from build123d import *

# Parameters (mm, degrees)
BOSS_EXTRUDE1_DEPTH = 3.175
CUT_EXTRUDE1_DEPTH  = 204.138678001
SKETCH3_W           = 42
SKETCH3_H           = 55.35
SKETCH3_W_2         = 7.65
SKETCH3_H_2         = 6.35
CUT_EXTRUDE2_DEPTH  = 204.138678001
SKETCH5_R           = 2
CUT_EXTRUDE4_DEPTH  = 204.138678001


with BuildPart() as part:
    # Sketch1 → Boss-Extrude1 (new, symmetric)
    with BuildSketch(Plane(origin=(0, 0, 0), x_dir=(1, 0, 0), z_dir=(0, 1, 0))):
        with BuildLine():
            Line((35, -200), (35, 0))
            ThreePointArc((35, 0), (0, 35), (-35, 0))
            Line((-35, 0), (-35, -200))
            Line((-35, -200), (35, -200))
        make_face()
    extrude(amount=BOSS_EXTRUDE1_DEPTH, both=True)

    # Sketch2 → Cut-Extrude1 (cut, through all)
    with BuildSketch(Plane(origin=(0, 3.175, 0), x_dir=(1, 0, 0), z_dir=(0, 1, 0))):
        with BuildLine():
            Line((-35, -38), (35, -38))
            Line((35, -38), (35, 0))
            ThreePointArc((35, 0), (0, 35), (-35, 0))
            Line((-35, 0), (-35, -38))
        make_face()
    extrude(amount=-CUT_EXTRUDE1_DEPTH, mode=Mode.SUBTRACT)

    # Sketch3 → Cut-Extrude2 (cut, through all)
    with BuildSketch(Plane(origin=(0, 3.175, 0), x_dir=(1, 0, 0), z_dir=(0, 1, 0))):
        with Locations((0, -87.325)):
            Rectangle(SKETCH3_W, SKETCH3_H)
        with Locations((-24.825, -111.825)):
            Rectangle(SKETCH3_W_2, SKETCH3_H_2)
        with Locations((24.825, -111.825)):
            Rectangle(SKETCH3_W_2, SKETCH3_H_2)
    extrude(amount=-CUT_EXTRUDE2_DEPTH, mode=Mode.SUBTRACT)

    # Sketch5 → Cut-Extrude4 (cut, through all)
    with BuildSketch(Plane(origin=(0, 3.175, 0), x_dir=(1, 0, 0), z_dir=(0, 1, 0))):
        with Locations(Location((27.5, -195.35, 0), (0, 0, 270))):
            Circle(SKETCH5_R)
        with Locations(Location((-27.5, -195.35, 0), (0, 0, 270))):
            Circle(SKETCH5_R)
        with Locations((15, -65.35)):
            Circle(SKETCH5_R)
        with Locations((-15, -65.35)):
            Circle(SKETCH5_R)
    extrude(amount=-CUT_EXTRUDE4_DEPTH, mode=Mode.SUBTRACT)


solid = part.part
Could you check a few things on this model? Use its own coordinates, in mm. A direction names the side the tool comes from. Give positions to 0.01 mm unless a question says otherwise; leave off trailing zeros. Write each loop counter-clockwise with the first axis right and the second up, starting at its lowest first coordinate (ties: lowest second). Pieces come first, ordered by that corner, then holes. Notation, with made-up numbers: (65, 5) -> (107, 5) arc R11 ccw to (107, 12) -> close; hole circle Ø10 at (81.25, -9). An arc over 180 degrees is marked (long way). Answer as a JSON object with one key per item and string values.
Q1. Which directions (+Z, -Z, +X, -X, +Y, -Y) give clear straight access to the entire face, cutting with the end or side of a thin tool? Please do faces 4 (the flat face through (0, 0, 200)), 5 (the flat face through (-25, 0, 108.65)).
Taken from the geometry:
{"face 4": "+Z, +X, -X, +Y, -Y", "face 5": "+Y, -Y"}
Q2. Please list where these lines run through material, in increasing order: L1, parallel to X at y = -1.5, z = 195.35; L2, parallel to Z at x = -22, y = 0.75; L3, parallel to Z at x = -4, y = 0.
Taken from the geometry:
{"L1": "x = -35 to -29.5, -25.5 to 25.5, 29.5 to 35", "L2": "z = 38 to 108.65, 115 to 200", "L3": "z = 38 to 59.65, 115 to 200"}
Q3. Suppose I cut it at B-B on x = 16.5. Write out the boundary of the cut face in (y, z) (3 decimals).
Taken from the geometry:
{"outline": "(-3.175, 38) -> (3.175, 38) -> (3.175, 59.65) -> (-3.175, 59.65) -> close; (-3.175, 115) -> (3.175, 115) -> (3.175, 200) -> (-3.175, 200) -> close"}
Q4. Suppose I cut it at A-A on z = 195.35. Write out the boundary of the cut face in (x, y) (3 decimals).
Taken from the geometry:
{"outline": "(-35, -3.175) -> (-29.5, -3.175) -> (-29.5, 3.175) -> (-35, 3.175) -> close; (-25.5, -3.175) -> (25.5, -3.175) -> (25.5, 3.175) -> (-25.5, 3.175) -> close; (29.5, -3.175) -> (35, -3.175) -> (35, 3.175) -> (29.5, 3.175) -> close"}
Q5. We'd pull the mould along X, two halves only. Please class faces 1 (the flat face through (0, 3.175, 118)), 2 (the flat face through (-35, 0, 118)), 3 (the flat face through (0, 0, 59.65)): released by +X, released by -X, zero draft, split by the parting line, or undercut.
Taken from the geometry:
{"face 1": "zero draft", "face 2": "released by -X", "face 3": "undercut"}
Q6. Suppose I cut it at C-C on y = -1.25. Write out the boundary of the cut face in (x, z), then the cut area to 3 significant figures.
Taken from the geometry:
{"outline": "(-35, 38) -> (35, 38) -> (35, 200) -> (-35, 200) -> close; hole circle Ø4 at (-27.5, 195.35); hole (-28.65, 108.65) -> (-21, 108.65) -> (-21, 59.65) -> (21, 59.65) -> (21, 108.65) -> (28.65, 108.65) -> (28.65, 115) -> (-28.65, 115) -> close; hole circle Ø4 at (27.5, 195.35)", "area": "8,890 mm²"}
